```python
from build123d import *

# Parameters (mm, degrees)
SKETCH1_R           = 76.2
SKETCH1_R_2         = 14.224
BOSS_EXTRUDE1_DEPTH = 3.81
SKETCH4_R           = 16
SKETCH4_R_2         = 11
BOSS_EXTRUDE5_DEPTH = 7
SKETCH5_R           = 11
SKETCH5_R_2         = 9.5
BOSS_EXTRUDE6_DEPTH = 0.762
SKETCH6_R           = 2.55
CUT_EXTRUDE1_DEPTH  = 109.303906208


with BuildPart() as part:
    # Sketch1 → Boss-Extrude1 (new body)
    with BuildSketch(Plane(origin=(0, 0, 0), x_dir=(1, 0, 0), z_dir=(0, 1, 0))):
        with Locations(Location((0, 0, 0), (0, 0, 90))):
            Circle(SKETCH1_R)
        with Locations(Location((-57.15, 0, 0), (0, 0, 90))):
            Circle(SKETCH1_R_2, mode=Mode.SUBTRACT)
        with Locations(Location((-46.235321229, 33.591927169, 0), (0, 0, 90))):
            Circle(SKETCH1_R_2, mode=Mode.SUBTRACT)
        with Locations(Location((-17.660321229, 54.352879906, 0), (0, 0, 90))):
            Circle(SKETCH1_R_2, mode=Mode.SUBTRACT)
        with Locations(Location((17.660321229, 54.352879906, 0), (0, 0, 90))):
            Circle(SKETCH1_R_2, mode=Mode.SUBTRACT)
        with Locations(Location((46.235321229, 33.591927169, 0), (0, 0, 90))):
            Circle(SKETCH1_R_2, mode=Mode.SUBTRACT)
        with Locations(Location((57.15, 0, 0), (0, 0, 90))):
            Circle(SKETCH1_R_2, mode=Mode.SUBTRACT)
        with Locations(Location((46.235321229, -33.591927169, 0), (0, 0, 90))):
            Circle(SKETCH1_R_2, mode=Mode.SUBTRACT)
        with Locations(Location((17.660321229, -54.352879906, 0), (0, 0, 90))):
            Circle(SKETCH1_R_2, mode=Mode.SUBTRACT)
        with Locations(Location((-17.660321229, -54.352879906, 0), (0, 0, 90))):
            Circle(SKETCH1_R_2, mode=Mode.SUBTRACT)
        with Locations(Location((-46.235321229, -33.591927169, 0), (0, 0, 90))):
            Circle(SKETCH1_R_2, mode=Mode.SUBTRACT)
    extrude(amount=BOSS_EXTRUDE1_DEPTH)

    # Sketch4 → Boss-Extrude5 (add)
    with BuildSketch(Plane(origin=(0, 3.81, 0), x_dir=(1, 0, 0), z_dir=(0, 1, 0))):
        with Locations(Location((0, 0, 0), (0, 0, 270))):
            Circle(SKETCH4_R)
        with Locations(Location((0, 0, 0), (0, 0, 270))):
            Circle(SKETCH4_R_2, mode=Mode.SUBTRACT)
    extrude(amount=BOSS_EXTRUDE5_DEPTH)

    # Sketch5 → Boss-Extrude6 (add)
    with BuildSketch(Plane(origin=(0, 3.81, 0), x_dir=(1, 0, 0), z_dir=(0, 1, 0))):
        with Locations(Location((0, 0, 0), (0, 0, 270))):
            Circle(SKETCH5_R)
        with Locations(Location((0, 0, 0), (0, 0, 90))):
            Circle(SKETCH5_R_2, mode=Mode.SUBTRACT)
    extrude(amount=BOSS_EXTRUDE6_DEPTH)

    # Sketch6 → Cut-Extrude1 (cut, through all)
    with BuildSketch(Plane.XZ):
        with Locations(Location((0, 0, 0), (0, 0, 270))):
            Circle(SKETCH6_R)
    extrude(amount=-CUT_EXTRUDE1_DEPTH, mode=Mode.SUBTRACT)


solid = part.part
```
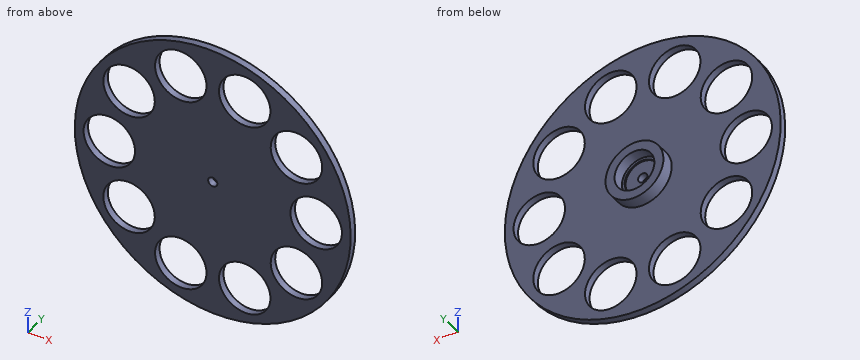
Design review of the part built by this model. Coordinates are the model's own, in mm. Coordinates: 2 decimals unless noted, no trailing zeros. Loops run counter-clockwise (first coordinate to the right, second up) from the corner with the lowest first, then second, coordinate; pieces in that order, holes last. Notation, with made-up numbers: (84, 35.25) -> (95, 35.25) arc R20 ccw to (95, 60.25) -> close; hole circle Ø2 at (-15.5, 38.25). An arc over 180 degrees is marked (long way). Answer as a JSON object with one key per item and string values.
Q1. Take a section at D-D on z = -29.5. Give the boundary of the cut face in (x, y).
Answer block:
{"outline": "(-70.26, 0) -> (-59.86, 0) -> (-59.86, 3.81) -> (-70.26, 3.81) -> close; (-32.61, 0) -> (32.61, 0) -> (32.61, 3.81) -> (-32.61, 3.81) -> close; (59.86, 0) -> (70.26, 0) -> (70.26, 3.81) -> (59.86, 3.81) -> close"}
Q2. Clearance check with flat-ended pins moving along their axes: pin 1 Ø6.5 at (x, z) = (0, 0) entering from +Y; pin 2 Ø1 at (x, y) = (-4.5, 5.5) entering from +Z; pin 3 Ø5 at (x, z) = (58.5, -32) entering from -Y; pin 4 Ø5 at (x, y) = (21, 2.5) entering from +Z. State where each tip first meets the part, or that it passes through.
Answer block:
{"pin 1": "stops at y = 3.81", "pin 2": "stops at z = 15.49", "pin 3": "stops at y = 0", "pin 4": "stops at z = 73.92"}
Q3. To check wall thickness, follow L1, parallel to X at y = 4.3, z = 0; L2, parallel to X at y = 1, z = -32; L3, parallel to Z at x = -58.5, y = 3.5. State the ranges of each line that lie inside material, in increasing order.
Answer block:
{"L1": "x = -16 to -9.5, 9.5 to 16", "L2": "x = -69.16 to -60.37, -32.1 to 32.1, 60.37 to 69.16", "L3": "z = -48.83 to -40.8, -26.39 to -14.16, 14.16 to 26.39, 40.8 to 48.83"}
Q4. Take a section at A-A on x = 0. Give the boundary of the cut face in (y, z), plus the area to 4 significant figures.
Answer block:
{"outline": "(0, -76.2) -> (3.81, -76.2) -> (3.81, -16) -> (10.81, -16) -> (10.81, -11) -> (4.57, -11) -> (4.57, -9.5) -> (3.81, -9.5) -> (3.81, -2.55) -> (0, -2.55) -> close; (0, 2.55) -> (3.81, 2.55) -> (3.81, 9.5) -> (4.57, 9.5) -> (4.57, 11) -> (10.81, 11) -> (10.81, 16) -> (3.81, 16) -> (3.81, 76.2) -> (0, 76.2) -> close", "area": "633.5 mm^2"}
Q5. Take a section at B-B on x = -57.15. Give the boundary of the cut face in (y, z).
Answer block:
{"outline": "(0, -50.4) -> (3.81, -50.4) -> (3.81, -42.71) -> (0, -42.71) -> close; (0, -24.47) -> (3.81, -24.47) -> (3.81, -14.22) -> (0, -14.22) -> close; (0, 14.22) -> (3.81, 14.22) -> (3.81, 24.47) -> (0, 24.47) -> close; (0, 42.71) -> (3.81, 42.71) -> (3.81, 50.4) -> (0, 50.4) -> close"}
Q6. Take a section at C-C on y = 8.75. Give the boundary of the cut face in (x, z), plus the area to 3 significant figures.
Answer block:
{"outline": "circle Ø32 at (0, 0); hole circle Ø22 at (0, 0)", "area": "424 mm^2"}
